Geometry: see drawing. Coordinates: mm, zero at the bounding-box minimum. A direction names the side the tool comes from. Round coordinates to 2 decimals unless told otherwise and drop trailing zeros. Loops run counter-clockwise (first coordinate to the right, second up) from the corner with the lowest first, then second, coordinate; pieces in that order, holes last. Notation, with made-up numbers: (35.25, -0.5) - (78.25, -0.5) arc R22 ccw to (78.25, 37.5) - close; hole circle Ø5 at (37.5, -2.5). An arc over 180 degrees is marked (long way). Answer in a Markdown table with one row per item. Add a question column.
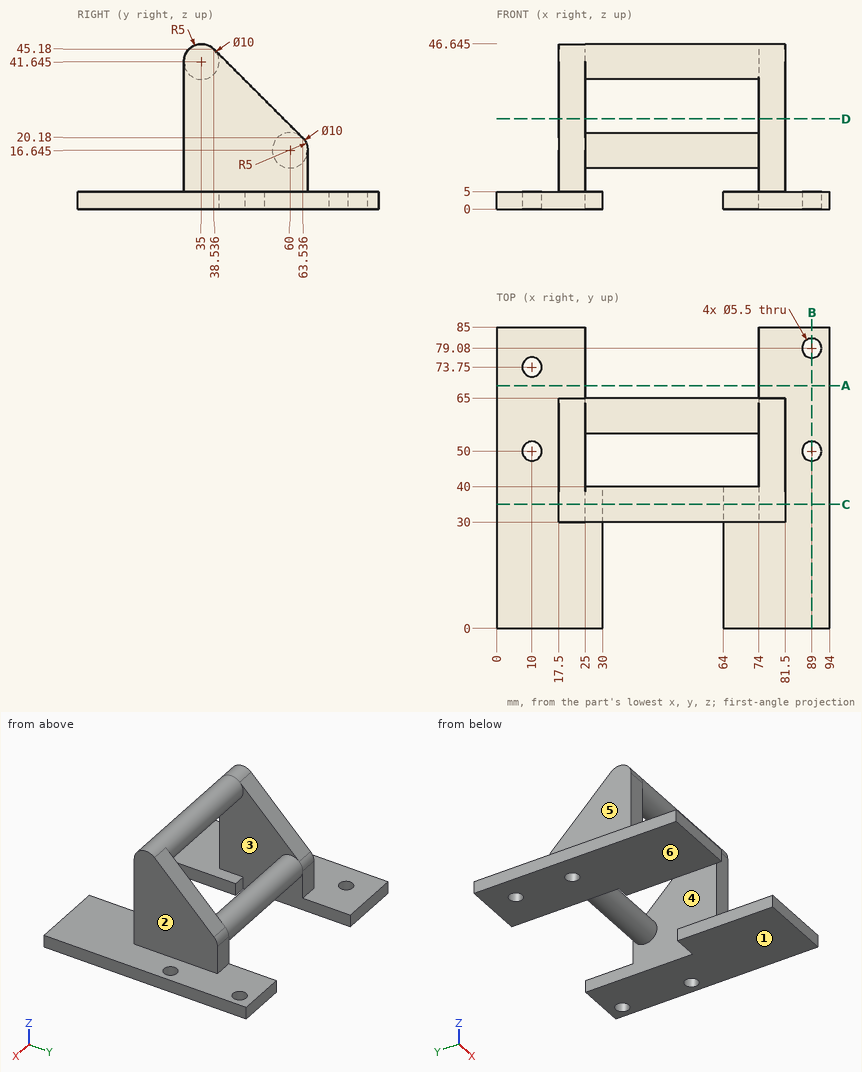
1) Reachability of the marked faces 4, 5 and 6 from +Z, -Z, +X, -X, +Y, -Y: full face, straight path, thin tool, end or side. Return the list, or none.
2) Material intervals for line 1 along Y through (x, z) = (89, 3); line 2 along X through (y, z) = (39, 3.5); line 3 along X through (y, z) = (32, 32.5), sorted ascending. Write a range as from..to.
3) Contact query for flat-ended pins moving along their axis: pin 1 Ø2.5 at (x, z) = (71, 3) entering from +Y; pin 2 Ø2 at (x, z) = (67.5, 19) entering from +Y; pin 3 Ø15 at (x, y) = (82.5, 22) entering from +Z; pin 4 Ø4 at (y, z) = (21, 1.5) entering from -X. Output: stop coordinate, or through.
4) Section D-D, the plane z = 25.5. Return the cut outline in (x, y) (1 decimal), and give its area (3 significant figures).
5) Pull-direction query (Z, two-part tool) for the marked faces 1, 2 and 3; classes: pulls with the +Z half, pulls with the -Z half, needs draft (parallel to the pull), parting line crosses it, or undercut.
6) Section A-A, the plane y = 68.5. Return the cut outline in (x, z), and give its area (3 significant figures).
7) Section C-C, the plane y = 35. Return the cut outline in (x, z) (1 decimal).
8) Section B-B, the plane x = 89. Return the cut outline in (y, z).
Evaluation:
| question | item | result |
|---|---|---|
| 1 | face 4 | none |
| 1 | face 5 | +Z, -X, +Y, -Y |
| 1 | face 6 | -Z, +X, -X, +Y, -Y |
| 2 | line 1 | y = 0..47.25, 52.75..76.33, 81.83..85 |
| 2 | line 2 | x = 0..30, 64..94 |
| 2 | line 3 | x = 17.5..25, 74..81.5 |
| 3 | pin 1 | stops at y = 40 |
| 3 | pin 2 | stops at y = 64.81 |
| 3 | pin 3 | stops at z = 5 |
| 3 | pin 4 | stops at x = 0 |
| 4 | outline | (17.5, 30) - (25, 30) - (25, 58.2) - (17.5, 58.2) - close; (74, 30) - (81.5, 30) - (81.5, 58.2) - (74, 58.2) - close |
| 4 | area | 423 mm² |
| 5 | face 1 | pulls with the -Z half |
| 5 | face 2 | needs draft |
| 5 | face 3 | undercut |
| 6 | outline | (0, 0) - (25, 0) - (25, 5) - (0, 5) - close; (74, 0) - (94, 0) - (94, 5) - (74, 5) - close |
| 6 | area | 225 mm² |
| 7 | outline | (0, 0) - (30, 0) - (30, 5) - (25, 5) - (25, 36.6) - (74, 36.6) - (74, 5) - (64, 5) - (64, 0) - (94, 0) - (94, 5) - (81.5, 5) - (81.5, 46.6) - (17.5, 46.6) - (17.5, 5) - (0, 5) - close |
| 8 | outline | (0, 0) - (47.25, 0) - (47.25, 5) - (0, 5) - close; (52.75, 0) - (76.33, 0) - (76.33, 5) - (52.75, 5) - close; (81.83, 0) - (85, 0) - (85, 5) - (81.83, 5) - close |
